Geometry check sheet. Reference: the model listing, model coordinates, mm. Face numbers are marked on the shaded views. Round coordinates to 2 decimals unless told otherwise and drop trailing zeros. Write each loop counter-clockwise with the first axis right and the second up, starting at its lowest first coordinate (ties: lowest second). Pieces come first, ordered by that corner, then holes.
Item 1: Scan lines: probe 1 along Y at (x, z) = (7, 5); probe 2 along Y at (x, z) = (-2, 4.5); probe 3 along Y at (x, z) = (-16.5, 6.5). Record each from-to range of solid material in increasing order.
Item 2: Cross-section at A-A (y = 0). Enter the section's corners in (x, z), then the cut area to 3 significant figures.
Item 3: Draft check along Y on the marked faces 1, 2, 3 and 4. Enter one of: pulls with the +Y half, pulls with the -Y half, needs draft (parallel to the pull), parting line crosses it, or undercut.
Item 4: Depth check by flat-ended pin: P1, Ø1.6, axis at y = 0.5, z = 5.5, coming from the -X side; P2, Ø4, axis at y = 0, z = 5, coming from the +X side; P3, Ø4, axis at x = -4, y = 7.5, coming from the -Z side. Enter the tip coordinate at first touch or a pass-through.
Item 5: Cross-section at B-B (z = 1.25). Enter the section's corners in (x, y).
from build123d import *

# Parameters (mm, degrees)
F0_R     = 22.5
F1_DEPTH = 2
F2_R     = 17.5
F3_DEPTH = 5
F5_DEPTH = 2
F6_R     = 1.5
F7_R     = 2
F8_R     = 16
F9_DEPTH = 6
F10_R    = 5.99999


# Not quite as in the source:
# - a fillet or chamfer is up to 0.001 mm smaller than in the source, because OpenCascade refuses the exact size


with BuildPart() as f1:
    # F0 (on Top) → F1 (new body)
    with BuildSketch(Plane.XY):
        Circle(F0_R)
    extrude(amount=F1_DEPTH)

    # F2 (on face) → F3 (join)
    with BuildSketch(Plane.XY.offset(2)):
        with Locations((0.8037949441, 0)):
            Circle(F2_R)
    extrude(amount=F3_DEPTH)

    # F4 (on face) → F5 (join)
    with BuildSketch(Plane.XY.offset(7)):
        with BuildLine():
            Line((-20.3037949441, -4), (-16.2329300933, -4))
            ThreePointArc((-16.2329300933, -4), (-16.6962050559, 0), (-16.2329300933, 4))
            Line((-16.2329300933, 4), (-20.3037949441, 4))
            Line((-20.3037949441, 4), (-20.3037949441, -4))
        make_face()
        with BuildLine():
            Line((-16.2329300933, -4), (17.8405199815, -4))
            ThreePointArc((17.8405199815, -4), (18.1875903893, -2.0133692962), (18.3037949441, 0))
            ThreePointArc((18.3037949441, 0), (18.1875903893, 2.0133692962), (17.8405199815, 4))
            Line((17.8405199815, 4), (-16.2329300933, 4))
            ThreePointArc((-16.2329300933, 4), (-16.6962050559, 0), (-16.2329300933, -4))
        make_face()
        with BuildLine():
            Line((17.8405199815, -4), (20.3037949441, -4))
            Line((20.3037949441, -4), (20.3037949441, 4))
            Line((20.3037949441, 4), (17.8405199815, 4))
            ThreePointArc((17.8405199815, 4), (18.1875903893, 2.0133692962), (18.3037949441, 0))
            ThreePointArc((18.3037949441, 0), (18.1875903893, -2.0133692962), (17.8405199815, -4))
        make_face()
    extrude(amount=-F5_DEPTH)

    # F6
    f6_edges = [f1.edges().sort_by_distance(p)[0] for p in [
        (18.18759, -2.013369, 5),
        (-16.696205, 0, 5),
        (18.18759, 2.013369, 5),
    ]]
    fillet(f6_edges, radius=F6_R)

    # F7
    f7_edges = [f1.edges().sort_by_distance(p)[0] for p in [
        (-20.303795, 4, 6),
        (-20.303795, -4, 6),
        (20.303795, -4, 6),
        (20.303795, 4, 6),
    ]]
    fillet(f7_edges, radius=F7_R)

    # F8 (on face) → F9 (cut)
    with BuildSketch(Plane(origin=(0, 0, 0), x_dir=(1, 0, 0), z_dir=(0, 0, -1))):
        Circle(F8_R)
    extrude(amount=-F9_DEPTH, mode=Mode.SUBTRACT)

    # F10 (radius 6 in the source; OpenCascade refuses exactly that, so slightly less here)
    f10_edges = [f1.edges().sort_by_distance(p)[0] for p in [
        (-16, 0, 6),
    ]]
    fillet(f10_edges, radius=F10_R)

    # F11 (on face) → F12 (join, up to the next surface of F1)
    with BuildSketch(Plane(origin=(0, 0, 0), x_dir=(1, 0, 0), z_dir=(0, 0, -1))):
        with BuildLine():
            Line((15.8034806293, 2.5), (-15.8034806293, 2.5))
            ThreePointArc((-15.8034806293, 2.5), (-16, 0), (-15.8034806293, -2.5))
            Line((-15.8034806293, -2.5), (15.8034806293, -2.5))
            ThreePointArc((15.8034806293, -2.5), (15.9507944954, -1.2538560387), (16, 0))
            ThreePointArc((16, 0), (15.9507944954, 1.2538560387), (15.8034806293, 2.5))
        make_face()
    extrude(until=Until.NEXT, dir=(0, 0, 1))


solid = f1.part
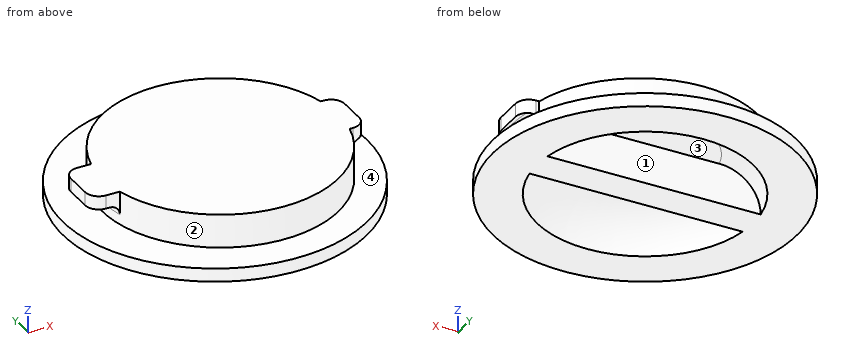
Resolved:
1. probe 1: y = -16.37 to -11.33, -2.5 to 2.5, 11.33 to 16.37
1. probe 2: y = -17.27 to -13.82, -2.5 to 2.5, 13.82 to 17.27
1. probe 3: y = -4 to 4
2. outline: (-22.5, 0) - (22.5, 0) - (22.5, 2) - (18.3, 2) - (18.3, 3.5) arc R1.5 cw to (19.8, 5) - (20.3, 5) - (20.3, 7) - (-20.3, 7) - (-20.3, 5) - (-18.2, 5) arc R1.5 cw to (-16.7, 3.5) - (-16.7, 2) - (-22.5, 2) - close
2. area: 277 mm2
3. face 1: undercut
3. face 2: parting line crosses it
3. face 3: undercut
3. face 4: needs draft
4. P1: stops at x = -20.3
4. P2: stops at x = 20.3
4. P3: stops at z = 5.98
5. outline: circle Ø45 at (0, 0); hole (-15.67, -2.5) arc R15.87 ccw to (15.67, -2.5) - close; hole (-15.67, 2.5) - (15.67, 2.5) arc R15.87 ccw to start
